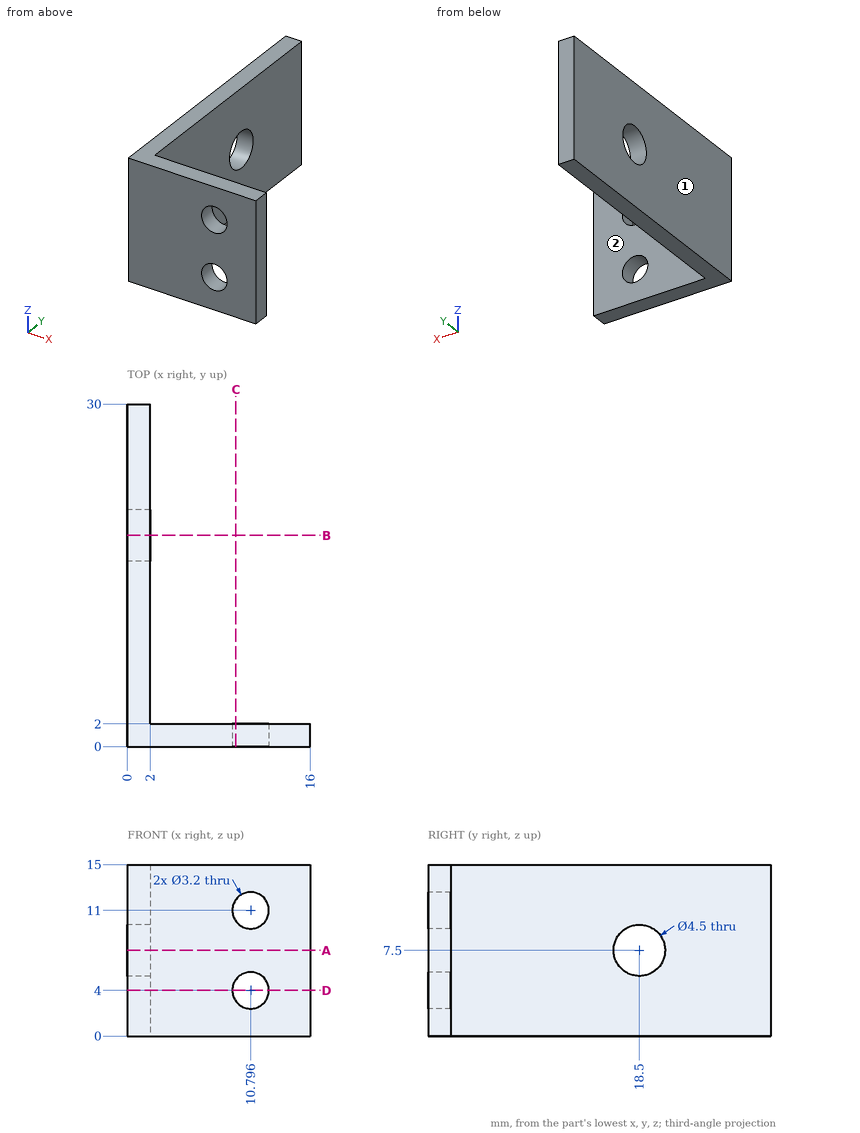
Source: three-view drawing plus pictorial views. Frame: mm from the lowest corner of the part. A direction names the side the tool comes from. Round coordinates to 2 decimals unless told otherwise and drop trailing zeros. Order: outer loops, then holes, each group sorted by start corner. A loop starts at its lowest first (then second) coordinate and runs counter-clockwise, first axis right, second up. Notation, with made-up numbers: (88, 12) -> (133, 12) arc R19 ccw to (133, 44) -> close; hole circle Ø10 at (3.5, 27.25). An arc over 180 degrees is marked (long way). Use CSV: the item, a comma, the result in double quotes. Start each with the question number.
1) Section D-D (z = 4). Return the cut outline in (x, y).
2) Section B-B (y = 18.5). Return the cut outline in (x, z), and give its area (3 significant figures).
3) Material intervals for line 1 along X through (y, z) = (1.6, 11); line 2 along Y through (x, z) = (4.25, 4.25), sorted ascending. Write a range as from..to.
4) First-contact query: pin 1 Ø2 at (y, z) = (27, 8.5) entering from +X; pin 2 Ø3.5 at (x, z) = (10.8, 11) entering from +Y. Flat tips, straight axial feed; report the tip coordinate or a pass-through.
5) Section A-A (z = 7.5). Return the cut outline in (x, y).
6) Set-up query: the marked faces 1 and 2. Return all of +Z, -Z, +X, -X, +Y, -Y with unobstructed straight access to the full face (end or side cutting, diameter ignored); none if empty.
7) Section C-C (x = 9.5). Return the cut outline in (y, z), and give its area (3 significant figures).
Returned:
1,outline,"(0, 0) -> (9.2, 0) -> (9.2, 2) -> (2, 2) -> (2, 30) -> (0, 30) -> close; (12.4, 0) -> (16, 0) -> (16, 2) -> (12.4, 2) -> close"
2,outline,"(0, 0) -> (2, 0) -> (2, 5.25) -> (0, 5.25) -> close; (0, 9.75) -> (2, 9.75) -> (2, 15) -> (0, 15) -> close"
2,area,"21.0 mm²"
3,line 1,"x = 0..9.2, 12.4..16"
3,line 2,"y = 0..2"
4,pin 1,"stops at x = 2"
4,pin 2,"stops at y = 2"
5,outline,"(0, 0) -> (16, 0) -> (16, 2) -> (2, 2) -> (2, 16.25) -> (0, 16.25) -> close; (0, 20.75) -> (2, 20.75) -> (2, 30) -> (0, 30) -> close"
6,face 1,"+Z, -Z, -X, +Y, -Y"
6,face 2,"+Z, -Z, +X, +Y"
7,outline,"(0, 0) -> (2, 0) -> (2, 3.06) -> (0, 3.06) -> close; (0, 4.94) -> (2, 4.94) -> (2, 10.06) -> (0, 10.06) -> close; (0, 11.94) -> (2, 11.94) -> (2, 15) -> (0, 15) -> close"
7,area,"22.5 mm²"
